Here's how the part is built. I have some questions about the finished solid (model axes, mm). A direction names the side the tool comes from. Round coordinates to 2 decimals unless told otherwise and drop trailing zeros. Loops run counter-clockwise (first coordinate to the right, second up) from the corner with the lowest first, then second, coordinate; pieces in that order, holes last. Notation, with made-up numbers: M 55.25,12 L 96.25,12 A31 ccw 96.25,38 Z; hole C -21,-10 d2. An arc over 180 degrees is marked long. Answer as a JSON object with one key per item and string values.
from build123d import *
from build123d.topology import SkipClean

# Parameters (mm, degrees)
SKETCH_1_R            = 1.35
SKETCH_1_R_2          = 5.1
SKETCH_1_R_3          = 6.1
EXTRUDE_1_DEPTH       = 5
EXTRUDE_START         = 1.5
SKETCH_1_4_R          = 6.1
SKETCH_1_4_R_2        = 5.1
SKETCH_1_4_R_3        = 2.1
EXTRUDE_3_DEPTH       = 2
FILLET_1_R            = 1
FILLET_2_R            = 1
FILLET_3_R            = 1
FILLET_4_R            = 1
FILLET_5_R            = 10
SKETCH_1_9_R          = 1.35
SKETCH_1_9_R_2        = 6.1
SKETCH_1_9_R_3        = 2.1
EXTRUDE_4_DEPTH       = 4
EXTRUDE_START_2       = 2
SKETCH_1_10_R         = 6.1
SKETCH_1_10_R_2       = 2.1
EXTRUDE_5_DEPTH       = 2
SKETCH_1_11_R         = 6.1
SKETCH_1_11_R_2       = 5.1
EXTRUDE_7_DEPTH       = 3.5
CUT_EXTRUDE_START     = 5
SKETCH_1_15_R         = 2.5
SKETCH_1_15_R_2       = 1.35
CUT_EXTRUDE_1_DEPTH   = 1
SKETCH_2_R            = 10
SKETCH_2_R_2          = 6.1
EXTRUDE_8_DEPTH       = 2
SKETCH_1_16_R         = 6.1
SKETCH_1_16_R_2       = 5.1
CUT_EXTRUDE_1_2_DEPTH = 1.5
SKETCH_3_R            = 6.1
SKETCH_3_R_2          = 5.1
EXTRUDE_9_DEPTH       = 1
CUT_EXTRUDE_2_DEPTH   = 1


with BuildPart() as part:
    # 草图1 → 凸台-拉伸1 (new body)
    with BuildSketch(Plane(origin=(0, 0, 0), x_dir=(1, 0, 0), z_dir=(0, 1, 0))):
        with BuildLine():
            Line((-105, 10), (-6.633249581, 10))
            ThreePointArc((-6.633249581, 10), (12, 0), (-6.633249581, -10))
            Line((-6.633249581, -10), (-105, -10))
            ThreePointArc((-105, -10), (-115, 0), (-105, 10))
        make_face()
        with Locations(Location((-5.656854249, 5.656854249, 0), (0, 0, 270))):
            Circle(SKETCH_1_R, mode=Mode.SUBTRACT)
        with Locations(Location((5.656854249, 5.656854249, 0), (0, 0, 270))):
            Circle(SKETCH_1_R, mode=Mode.SUBTRACT)
        with Locations(Location((5.656854249, -5.656854249, 0), (0, 0, 270))):
            Circle(SKETCH_1_R, mode=Mode.SUBTRACT)
        with Locations(Location((-5.656854249, -5.656854249, 0), (0, 0, 270))):
            Circle(SKETCH_1_R, mode=Mode.SUBTRACT)
        with Locations(Location((0, 0, 0), (0, 0, 270))):
            Circle(SKETCH_1_R_2, mode=Mode.SUBTRACT)
        with Locations(Location((-105, 0, 0), (0, 0, 270))):
            Circle(SKETCH_1_R_3, mode=Mode.SUBTRACT)
        Polygon((-90.303388877, -5), (-45.422080483, -5), (-67.86273468, 2.88027015), align=None, mode=Mode.SUBTRACT)
        with BuildLine():
            Line((-96.339745962, 5), (-73.899091765, 5))
            Line((-73.899091765, 5), (-95.323626495, -2.523449184))
            ThreePointArc((-95.323626495, -2.523449184), (-95.08997733, 1.33845085), (-96.339745962, 5))
        make_face(mode=Mode.SUBTRACT)
        Polygon((-61.826377594, 5), (-39.385723397, -2.88027015), (-16.9450692, 5), align=None, mode=Mode.SUBTRACT)
        with BuildLine():
            Line((-33.349366312, -5), (-11.715632737, 2.596911544))
            ThreePointArc((-11.715632737, 2.596911544), (-11.93287523, -1.267473374), (-10.908712115, -5))
            Line((-10.908712115, -5), (-33.349366312, -5))
        make_face(mode=Mode.SUBTRACT)
    extrude(amount=EXTRUDE_1_DEPTH)

    # 草图1<4> → 凸台-拉伸3 (add)
    # profile 1 of 2: a face of its own
    with BuildSketch(Plane(origin=(0, 0, 0), x_dir=(1, 0, 0), z_dir=(0, 1, 0)).offset(EXTRUDE_START)):
        Circle(SKETCH_1_4_R)
        with Locations(Location((0, 0, 0), (0, 0, 270))):
            Circle(SKETCH_1_4_R_2, mode=Mode.SUBTRACT)
    # profile 2 of 2: a face of its own
    with BuildSketch(Plane(origin=(0, 0, 0), x_dir=(1, 0, 0), z_dir=(0, 1, 0)).offset(EXTRUDE_START)):
        with Locations(Location((0, 0, 0), (0, 0, 270))):
            Circle(SKETCH_1_4_R_2)
        with Locations(Location((0, 0, 0), (0, 0, 270))):
            Circle(SKETCH_1_4_R_3, mode=Mode.SUBTRACT)
    extrude(amount=EXTRUDE_3_DEPTH)

    # 圆角1
    fillet_1_edges = [part.edges().sort_by_distance(p)[0] for p in [
        (-73.899091765, 2.5, -5),
        (-96.339745962, 2.5, -5),
        (-95.323626495, 2.5, 2.523449184),
    ]]
    fillet(fillet_1_edges, radius=FILLET_1_R)

    # 圆角2
    fillet_2_edges = [part.edges().sort_by_distance(p)[0] for p in [
        (-90.303388877, 2.5, 5),
        (-45.422080483, 2.5, 5),
        (-67.86273468, 2.5, -2.88027015),
    ]]
    fillet(fillet_2_edges, radius=FILLET_2_R)

    # 圆角3
    fillet_3_edges = [part.edges().sort_by_distance(p)[0] for p in [
        (-39.385723397, 2.5, 2.88027015),
        (-16.9450692, 2.5, -5),
        (-61.826377594, 2.5, -5),
    ]]
    fillet(fillet_3_edges, radius=FILLET_3_R)

    # 圆角4
    fillet_4_edges = [part.edges().sort_by_distance(p)[0] for p in [
        (-33.349366312, 2.5, 5),
        (-10.908712115, 2.5, 5),
        (-11.715632737, 2.5, -2.596911544),
    ]]
    fillet(fillet_4_edges, radius=FILLET_4_R)

    # 圆角5
    fillet_5_edges = [part.edges().sort_by_distance(p)[0] for p in [
        (-6.633249581, 2.5, -10),
        (-6.633249581, 2.5, 10),
    ]]
    fillet(fillet_5_edges, radius=FILLET_5_R)

    # 草图1<9> → 凸台-拉伸4 (add)
    # profile 1 of 2: a face of its own
    with BuildSketch(Plane(origin=(0, 0, 0), x_dir=(1, 0, 0), z_dir=(0, 1, 0))):
        with BuildLine():
            Line((-105, 10), (-6.633249581, 10))
            ThreePointArc((-6.633249581, 10), (12, 0), (-6.633249581, -10))
            Line((-6.633249581, -10), (-105, -10))
            ThreePointArc((-105, -10), (-115, 0), (-105, 10))
        make_face()
        with Locations(Location((-5.656854249, 5.656854249, 0), (0, 0, 270))):
            Circle(SKETCH_1_9_R, mode=Mode.SUBTRACT)
        with Locations(Location((5.656854249, 5.656854249, 0), (0, 0, 270))):
            Circle(SKETCH_1_9_R, mode=Mode.SUBTRACT)
        with Locations(Location((5.656854249, -5.656854249, 0), (0, 0, 270))):
            Circle(SKETCH_1_9_R, mode=Mode.SUBTRACT)
        with Locations(Location((-5.656854249, -5.656854249, 0), (0, 0, 270))):
            Circle(SKETCH_1_9_R, mode=Mode.SUBTRACT)
        with Locations(Location((-105, 0, 0), (0, 0, 270))):
            Circle(SKETCH_1_9_R_2, mode=Mode.SUBTRACT)
        Circle(SKETCH_1_9_R_2, mode=Mode.SUBTRACT)
        Polygon((-90.303388877, -5), (-45.422080483, -5), (-67.86273468, 2.88027015), align=None, mode=Mode.SUBTRACT)
        with BuildLine():
            Line((-96.339745962, 5), (-73.899091765, 5))
            Line((-73.899091765, 5), (-95.323626495, -2.523449184))
            ThreePointArc((-95.323626495, -2.523449184), (-95.08997733, 1.33845085), (-96.339745962, 5))
        make_face(mode=Mode.SUBTRACT)
        Polygon((-61.826377594, 5), (-39.385723397, -2.88027015), (-16.9450692, 5), align=None, mode=Mode.SUBTRACT)
        with BuildLine():
            Line((-33.349366312, -5), (-11.715632737, 2.596911544))
            ThreePointArc((-11.715632737, 2.596911544), (-11.93287523, -1.267473374), (-10.908712115, -5))
            Line((-10.908712115, -5), (-33.349366312, -5))
        make_face(mode=Mode.SUBTRACT)
    # profile 2 of 2: a face of its own
    with BuildSketch(Plane(origin=(0, 0, 0), x_dir=(1, 0, 0), z_dir=(0, 1, 0))):
        with Locations((-105, 0)):
            Circle(SKETCH_1_9_R_3)
    extrude(amount=EXTRUDE_4_DEPTH)


with BuildPart() as extrude_4_kept_piece:
    # of the separate pieces the step leaves, the one the design keeps (extrude_4_pieces_kept)
    add(part.part.solids().sort_by_distance((-9.16515139, 0, 10))[0])

    # 草图1<10> → 凸台-拉伸5 (add)
    with BuildSketch(Plane(origin=(0, 0, 0), x_dir=(1, 0, 0), z_dir=(0, 1, 0)).offset(EXTRUDE_START_2)):
        with Locations(Location((-105, 0, 0), (0, 0, 270))):
            Circle(SKETCH_1_10_R)
        with Locations(Location((-105, 0, 0), (0, 0, 270))):
            Circle(SKETCH_1_10_R_2, mode=Mode.SUBTRACT)
    extrude(amount=EXTRUDE_5_DEPTH)

    # 草图1<11> → 凸台-拉伸7 (add)
    with BuildSketch(Plane(origin=(0, 0, 0), x_dir=(1, 0, 0), z_dir=(0, 1, 0))):
        Circle(SKETCH_1_11_R)
        with Locations(Location((0, 0, 0), (0, 0, 270))):
            Circle(SKETCH_1_11_R_2, mode=Mode.SUBTRACT)
    extrude(amount=EXTRUDE_7_DEPTH)

    # 草图1<15> → Cut-Extrude 1 (cut)
    # profile 1 of 4: a face of its own
    with BuildSketch(Plane(origin=(0, 0, 0), x_dir=(1, 0, 0), z_dir=(0, 1, 0)).offset(CUT_EXTRUDE_START)):
        with Locations((-5.656854249, 5.656854249)):
            Circle(SKETCH_1_15_R)
        with Locations((-5.656854249, 5.656854249)):
            Circle(SKETCH_1_15_R_2, mode=Mode.SUBTRACT)
    # profile 2 of 4: a face of its own
    with BuildSketch(Plane(origin=(0, 0, 0), x_dir=(1, 0, 0), z_dir=(0, 1, 0)).offset(CUT_EXTRUDE_START)):
        with Locations((5.656854249, 5.656854249)):
            Circle(SKETCH_1_15_R)
        with Locations((5.656854249, 5.656854249)):
            Circle(SKETCH_1_15_R_2, mode=Mode.SUBTRACT)
    # profile 3 of 4: a face of its own
    with BuildSketch(Plane(origin=(0, 0, 0), x_dir=(1, 0, 0), z_dir=(0, 1, 0)).offset(CUT_EXTRUDE_START)):
        with Locations((5.656854249, -5.656854249)):
            Circle(SKETCH_1_15_R)
        with Locations((5.656854249, -5.656854249)):
            Circle(SKETCH_1_15_R_2, mode=Mode.SUBTRACT)
    # profile 4 of 4: a face of its own
    with BuildSketch(Plane(origin=(0, 0, 0), x_dir=(1, 0, 0), z_dir=(0, 1, 0)).offset(CUT_EXTRUDE_START)):
        with Locations((-5.656854249, -5.656854249)):
            Circle(SKETCH_1_15_R)
        with Locations((-5.656854249, -5.656854249)):
            Circle(SKETCH_1_15_R_2, mode=Mode.SUBTRACT)
    extrude(amount=-CUT_EXTRUDE_1_DEPTH, mode=Mode.SUBTRACT)

    # 草图2 → 凸台-拉伸8 (add)
    with SkipClean():  # the faces are left unmerged after this step: merging them gives an invalid solid
        with BuildSketch(Plane.XZ):
            with Locations(Location((-105, 0, 0), (0, 0, 270))):
                Circle(SKETCH_2_R)
            with Locations(Location((-105, 0, 0), (0, 0, 270))):
                Circle(SKETCH_2_R_2, mode=Mode.SUBTRACT)
        extrude(amount=EXTRUDE_8_DEPTH)

    # 草图1<16> → Cut-Extrude 1 2 (cut)
    with SkipClean():  # the faces are left unmerged after this step: merging them gives an invalid solid
        with BuildSketch(Plane(origin=(0, 0, 0), x_dir=(1, 0, 0), z_dir=(0, 1, 0))):
            with Locations(Location((0, 0, 0), (0, 0, 270))):
                Circle(SKETCH_1_16_R)
            with Locations(Location((0, 0, 0), (0, 0, 270))):
                Circle(SKETCH_1_16_R_2, mode=Mode.SUBTRACT)
        extrude(amount=CUT_EXTRUDE_1_2_DEPTH, mode=Mode.SUBTRACT)

    # 草图3 → 凸台-拉伸9 (add)
    with SkipClean():  # the faces are left unmerged after this step: merging them gives an invalid solid
        with BuildSketch(Plane(origin=(0, 5, 0), x_dir=(1, 0, 0), z_dir=(0, 1, 0))):
            with Locations(Location((-105, 0, 0), (0, 0, 90))):
                Circle(SKETCH_3_R)
            with Locations(Location((-105, 0, 0), (0, 0, 270))):
                Circle(SKETCH_3_R_2, mode=Mode.SUBTRACT)
        extrude(amount=-EXTRUDE_9_DEPTH)

    # 草图4 → 切除-拉伸2 (cut)
    with SkipClean():  # the faces are left unmerged after this step: merging them gives an invalid solid
        with BuildSketch(Plane.XZ.offset(-1.5)):
            Polygon((3.983716857, 0), (1.991858429, 3.45), (-1.991858429, 3.45), (-3.983716857, 0), (-1.991858429, -3.45), (1.991858429, -3.45), align=None)
        extrude(amount=-CUT_EXTRUDE_2_DEPTH, mode=Mode.SUBTRACT)


solid = extrude_4_kept_piece.part
Item 1: I want a section at B-B on x = -75. List the corners of the cut face in (y, z) for me.
Solution:
{"outline": "M 0,-10 L 5,-10 L 5,-0.37 L 0,-0.37 Z; M 0,5 L 5,5 L 5,10 L 0,10 Z"}
Item 2: If I drill on L1, parallel to Z at x = 0, y = 3; L2, parallel to Y at x = -44, z = 6.25; L3, parallel to X at y = 3, z = 6.5, over which ranges is the centre line in solid material (lowest first)? Write a range as from..to.
Solution:
{"L1": "z = -12..-2.1, 2.1..12", "L2": "y = 0..5", "L3": "x = -112.6..-6.71, -4.6..4.6, 6.71..10.09"}
Item 3: For P1, Ø4.5, axis at x = 5.66, z = 5.66, coming from the +Y side; P2, Ø11, axis at x = -2, z = -0.5, coming from the -Y side; P3, Ø8, axis at x = -105, z = 0, coming from the -Y side; P4, Ø4, axis at x = 0, z = 0, coming from the +Y side, each with a flat end and sliding along its axis, tell me the tip position at first contact or that it passes through.
Solution:
{"P1": "stops at y = 4", "P2": "stops at y = 0", "P3": "stops at y = 2", "P4": "passes through"}
Item 4: I want a section at C-C on x = -89.5. List the corners of the cut face in (y, z) for me.
Solution:
{"outline": "M 0,-10 L 5,-10 L 5,-5 L 0,-5 Z; M 0,0.48 L 5,0.48 L 5,10 L 0,10 Z"}
Item 5: I want a section at A-A on x = 0. List the corners of the cut face in (y, z) for me, plus the area to 3 significant figures.
Solution:
{"outline": "M 0,-12 L 5,-12 L 5,-5.1 L 3.5,-5.1 L 3.5,-2.1 L 2.5,-2.1 L 2.5,-3.45 L 1.5,-3.45 L 1.5,-6.1 L 0,-6.1 Z; M 0,6.1 L 1.5,6.1 L 1.5,3.45 L 2.5,3.45 L 2.5,2.1 L 3.5,2.1 L 3.5,5.1 L 5,5.1 L 5,12 L 0,12 Z", "area": "75.3 mm2"}
Item 6: We'd pull the mould along Z, two halves only. Please class faces 1 (the face through (-78.783, 2.535, -4.187)), 2 (the face through (-7.063, 2.535, -10.224)), 3 (the face through (12, 2, 0)): +Z half, -Z half, draft (parallel to the pull), parting line (faces both ways), or undercut.
Solution:
{"face 1": "undercut", "face 2": "-Z half", "face 3": "parting line"}
Item 7: For faces 4 (the face through (-76.365, 2.465, 0.106)), 5 (the face through (2, 2.5, 2)), 6 (the face through (-107.2, 4, 1.1)), which set-ups out of +Z, -Z, +X, -X, +Y, -Y let a thin tool reach every point of the face, with its end or its side?
Solution:
{"face 4": "+Y, -Y", "face 5": "-Y", "face 6": "+Y"}
